Study the drawing (mm; zero at the part's minimum x, y, z) and answer. Coordinates: 2 decimals unless noted, no trailing zeros. Order: outer loops, then holes, each group sorted by start corner. A loop starts at its lowest first (then second) coordinate and runs counter-clockwise, first axis right, second up. Notation, with made-up numbers: M 65.5,52 L 92.5,52 A25 cw 92.5,78 Z; hole C -20,27.5 d4. An arc over 180 degrees is marked long. Put each result on its own line as item: value.
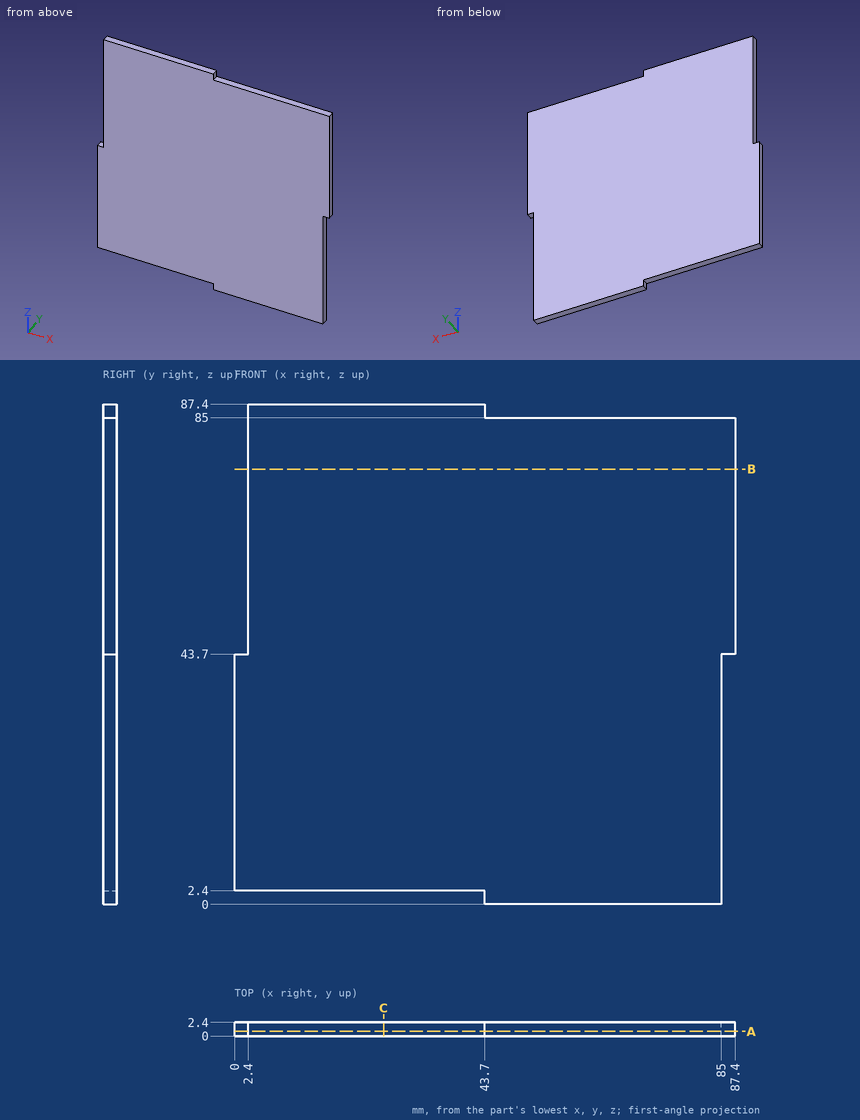
Q1. Find section A-A on y = 0.8. Write down the section's boundary in (x, z).
Answers below:
outline: M 0,2.4 L 43.7,2.4 L 43.7,0 L 85,0 L 85,43.7 L 87.4,43.7 L 87.4,85 L 43.7,85 L 43.7,87.4 L 2.4,87.4 L 2.4,43.7 L 0,43.7 Z
Q2. Consider line 1 along Z through (x, y) = (77, 0.15); line 2 along Z through (x, y) = (11.5, 1.5). Determine where each line is inside the solid, lowest interval first.
Answers below:
line 1: z = 0 to 85
line 2: z = 2.4 to 87.4
Q3. Find section C-C on x = 26. Write down the section's boundary in (y, z).
Answers below:
outline: M 0,2.4 L 2.4,2.4 L 2.4,87.4 L 0,87.4 Z
Q4. Given pin 1 (1.2 mm diameter, centred on x = 1, y = 1, fed in from +Z); pin 2 (1 mm diameter, centred on y = 1.5, z = 31.5, fed in from +X); pin 3 (0.7 mm diameter, centred on x = 86.5, y = 1.5, fed in from -Z), each flat-ended and moving along its own axis, determine where each tip first touches the part or whether it passes through.
Answers below:
pin 1: stops at z = 43.7
pin 2: stops at x = 85
pin 3: stops at z = 43.7
Q5. Find section B-B on z = 76. Write down the section's boundary in (x, y), plus the area to 3 significant figures.
Answers below:
outline: M 2.4,0 L 87.4,0 L 87.4,2.4 L 2.4,2.4 Z
area: 204 mm^2
